Check sheet for the modelled part. Datum: model origin and axes. Units: mm. Face numbers are marked on the shaded views. Round coordinates to 2 decimals unless told otherwise and drop trailing zeros. Write each loop counter-clockwise with the first axis right and the second up, starting at its lowest first coordinate (ties: lowest second). Pieces come first, ordered by that corner, then holes. Notation, with made-up numbers: (-0.75, 86) -> (20.25, 86) arc R21 ccw to (20.25, 94) -> close; hole circle Ø11 at (79, 89). An arc over 180 degrees is marked (long way). Answer as a JSON object with one key per item and string values. Group by question number.
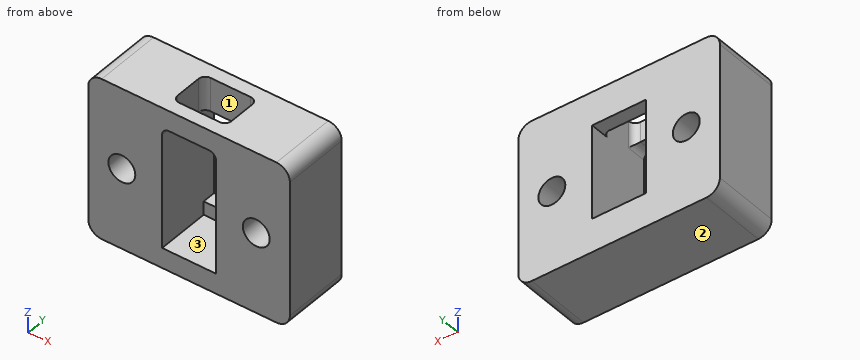
```python
from build123d import *

# Parameters (mm, degrees)
SKETCH1_W           = 38.1
SKETCH1_H           = 30.48
SKETCH1_R           = 2.54
SKETCH1_W_2         = 10.16
SKETCH1_H_2         = 22.86
BOSS_EXTRUDE1_DEPTH = 12.7
SKETCH2_W           = 10.16
SKETCH2_H           = 2.54
BOSS_EXTRUDE2_DEPTH = 2.54
SKETCH3_W           = 10.16
SKETCH3_H           = 2.54
BOSS_EXTRUDE3_DEPTH = 2.54
FILLET1_R           = 2.54
SKETCH4_W           = 10.16
SKETCH4_H           = 7.62
CUT_EXTRUDE1_DEPTH  = 36.149415358
FILLET2_R           = 1.27


with BuildPart() as part:
    # Sketch1 → Boss-Extrude1 (new body)
    with BuildSketch(Plane(origin=(0, 0, 0), x_dir=(1, 0, 0), z_dir=(0, 1, 0))):
        Rectangle(SKETCH1_W, SKETCH1_H)
        with Locations(Location((12.7, 0, 0), (0, 0, 270))):
            Circle(SKETCH1_R, mode=Mode.SUBTRACT)
        with Locations(Location((-12.7, 0, 0), (0, 0, 270))):
            Circle(SKETCH1_R, mode=Mode.SUBTRACT)
        Rectangle(SKETCH1_W_2, SKETCH1_H_2, mode=Mode.SUBTRACT)
    extrude(amount=-BOSS_EXTRUDE1_DEPTH)

    # Sketch2 → Boss-Extrude2 (add)
    with BuildSketch(Plane.XY.offset(-11.43)):
        with Locations((0, -1.27)):
            Rectangle(SKETCH2_W, SKETCH2_H)
    extrude(amount=BOSS_EXTRUDE2_DEPTH)

    # Sketch3 → Boss-Extrude3 (add)
    with BuildSketch(Plane(origin=(0, 0, 11.43), x_dir=(-1, 0, 0), z_dir=(0, 0, -1))):
        with Locations((0, -1.27)):
            Rectangle(SKETCH3_W, SKETCH3_H)
    extrude(amount=BOSS_EXTRUDE3_DEPTH)

    # Fillet1
    fillet1_edges = [part.edges().sort_by_distance(p)[0] for p in [
        (19.05, -6.35, 15.24),
        (-19.05, -6.35, 15.24),
        (-19.05, -6.35, -15.24),
        (19.05, -6.35, -15.24),
    ]]
    fillet(fillet1_edges, radius=FILLET1_R)

    # Sketch4 → Cut-Extrude1 (cut, through all)
    with BuildSketch(Plane(origin=(0, 0, 11.43), x_dir=(-1, 0, 0), z_dir=(0, 0, -1))):
        with Locations((0, -6.35)):
            Rectangle(SKETCH4_W, SKETCH4_H)
    extrude(amount=-CUT_EXTRUDE1_DEPTH, mode=Mode.SUBTRACT)

    # Fillet2
    fillet2_edges = [part.edges().sort_by_distance(p)[0] for p in [
        (-5.08, -11.43, 11.43),
        (5.08, -11.43, 11.43),
        (-5.08, -2.54, 12.065),
        (5.08, -2.54, 12.065),
        (5.08, -10.16, 13.335),
        (-5.08, -10.16, 13.335),
    ]]
    fillet(fillet2_edges, radius=FILLET2_R)


solid = part.part
```
(1) Section check D-D on z = -6. Record the cut outline in (x, y), then the cut area to 3 significant figures.
(2) Section check B-B on x = 12.7. Record the cut outline in (y, z), then the cut area to 3 significant figures.
(3) Section check A-A on z = 0. Record the cut outline in (x, y).
(4) Go/stop test with flat-tipped pins: pin 1 Ø3 at (x, z) = (12.7, 0) entering from -Y; pin 2 Ø1.3 at (x, z) = (-2, -10) entering from -Y. Record where each tip stops, or that it passes through.
(5) Section check C-C on y = -11. Record the cut outline in (x, z), then the cut area to 3 significant figures.
(6) Release check for a two-part mould opening along Z. For the marked faces 1, 2 and 3 record: pulls with the +Z half, pulls with the -Z half, needs draft (parallel to the pull), parting line crosses it, or undercut.
(7) Scan lines: line 1 along X through (y, z) = (-2.75, 0); line 2 along Y through (x, z) = (2.5, 12); line 3 along X through (y, z) = (-12, -8). Record each from-to range of solid material in increasing order.
Data:
{
 "1": {"outline": "(-19.05, -12.7) -> (-5.08, -12.7) -> (-5.08, 0) -> (-19.05, 0) -> close; (5.08, -12.7) -> (19.05, -12.7) -> (19.05, 0) -> (5.08, 0) -> close", "area": "355 mm²"},
 "2": {"outline": "(-12.7, -15.24) -> (0, -15.24) -> (0, -2.54) -> (-12.7, -2.54) -> close; (-12.7, 2.54) -> (0, 2.54) -> (0, 15.24) -> (-12.7, 15.24) -> close", "area": "323 mm²"},
 "3": {"outline": "(-19.05, -12.7) -> (-15.24, -12.7) -> (-15.24, 0) -> (-19.05, 0) -> close; (-10.16, -12.7) -> (-5.08, -12.7) -> (-5.08, 0) -> (-10.16, 0) -> close; (5.08, -12.7) -> (10.16, -12.7) -> (10.16, 0) -> (5.08, 0) -> close; (15.24, -12.7) -> (19.05, -12.7) -> (19.05, 0) -> (15.24, 0) -> close"},
 "4": {"pin 1": "passes through", "pin 2": "stops at y = -2.54"},
 "5": {"outline": "(-19.05, -12.7) arc R2.54 ccw to (-16.51, -15.24) -> (16.51, -15.24) arc R2.54 ccw to (19.05, -12.7) -> (19.05, 12.7) arc R2.54 ccw to (16.51, 15.24) -> (-16.51, 15.24) arc R2.54 ccw to (-19.05, 12.7) -> close; hole circle Ø5.08 at (-12.7, 0); hole (-5.08, -11.43) -> (5.08, -11.43) -> (5.08, 10.16) arc R1.27 ccw to (3.81, 11.43) -> (-3.81, 11.43) arc R1.27 ccw to (-5.08, 10.16) -> close; hole circle Ø5.08 at (12.7, 0)", "area": "884 mm²"},
 "6": {"face 1": "needs draft", "face 2": "pulls with the -Z half", "face 3": "undercut"},
 "7": {"line 1": "x = -19.05 to -15.24, -10.16 to -5.08, 5.08 to 10.16, 15.24 to 19.05", "line 2": "y = -12.7 to -10.16, -2.54 to 0", "line 3": "x = -19.05 to -5.08, 5.08 to 19.05"}
}
